Build history of the part. All positions in model axes, mm. Face numbers are marked on the shaded views. Round coordinates to 2 decimals unless told otherwise and drop trailing zeros. Order: outer loops, then holes, each group sorted by start corner. A loop starts at its lowest first (then second) coordinate and runs counter-clockwise, first axis right, second up. Notation, with made-up numbers: (-8.75, 17.5) -> (46.25, 17.5) arc R33 ccw to (46.25, 46.5) -> close; hole circle Ø9 at (81.5, -8.75). An arc over 180 degrees is marked (long way). Write item = value, one per line.
from build123d import *

# Parameters (mm, degrees)
SKETCH1_W             = 152.4
SKETCH1_H             = 101.6
BOSS_EXTRUDE2_DEPTH   = 6.35
SKETCH2_W             = 6.35
SKETCH2_H             = 12.7
SKETCH2_H_2           = 6.35
CUT_EXTRUDE2_DEPTH    = 6.35
SKETCH2_4_W           = 12.7
SKETCH2_4_H           = 6.35
CUT_EXTRUDE3_DEPTH    = 6.35
F_5_0MM_DOWEL_HOLE7_D = 5.3


with BuildPart() as part:
    # Sketch1 → Boss-Extrude2 (new body)
    with BuildSketch(Plane(origin=(0, 0, 0), x_dir=(1, 0, 0), z_dir=(0, 1, 0))):
        with Locations((76.2, 50.8)):
            Rectangle(SKETCH1_W, SKETCH1_H)
    extrude(amount=BOSS_EXTRUDE2_DEPTH)

    # Sketch2 → Cut-Extrude2 (cut)
    with BuildSketch(Plane(origin=(0, 6.35, 0), x_dir=(1, 0, 0), z_dir=(0, 1, 0))):
        with Locations((3.175, 19.05)):
            Rectangle(SKETCH2_W, SKETCH2_H)
        with Locations((3.175, 44.45)):
            Rectangle(SKETCH2_W, SKETCH2_H)
        with Locations((3.175, 69.85)):
            Rectangle(SKETCH2_W, SKETCH2_H)
        with Locations((3.175, 98.425)):
            Rectangle(SKETCH2_W, SKETCH2_H_2)
        with Locations((3.175, 92.075)):
            Rectangle(SKETCH2_W, SKETCH2_H_2)
    cut_extrude2 = extrude(amount=-CUT_EXTRUDE2_DEPTH, mode=Mode.SUBTRACT)

    # Mirror1: Cut-Extrude2 across plane
    add(cut_extrude2.mirror(Plane.ZY.offset(-76.2)), mode=Mode.SUBTRACT)

    # Sketch2_4 → Cut-Extrude3 (cut)
    with BuildSketch(Plane(origin=(0, 6.35, 0), x_dir=(1, 0, 0), z_dir=(0, 1, 0))):
        with Locations((19.05, 98.425)):
            Rectangle(SKETCH2_4_W, SKETCH2_4_H)
        with Locations((44.45, 98.425)):
            Rectangle(SKETCH2_4_W, SKETCH2_4_H)
        with Locations((69.85, 98.425)):
            Rectangle(SKETCH2_4_W, SKETCH2_4_H)
        with Locations((95.25, 98.425)):
            Rectangle(SKETCH2_4_W, SKETCH2_4_H)
        with Locations((146.05, 98.425)):
            Rectangle(SKETCH2_4_W, SKETCH2_4_H)
        with Locations((120.65, 98.425)):
            Rectangle(SKETCH2_4_W, SKETCH2_4_H)
    cut_extrude3 = extrude(amount=-CUT_EXTRUDE3_DEPTH, mode=Mode.SUBTRACT)

    # Mirror2: Cut-Extrude3 across plane
    add(cut_extrude3.mirror(Plane(origin=(0, 0, -50.8), x_dir=(1, 0, 0), z_dir=(0, 0, -1))), mode=Mode.SUBTRACT)

    # 5.0mm Dowel Hole7 (through all)
    with Locations(Plane(origin=(0, 0, 0), x_dir=(-1, 0, 0), z_dir=(0, -1, 0))):
        with Locations((-119.634, 79.65), (-32.766, 79.65), (-32.766, 21.95), (-119.634, 21.95)):
            Hole(F_5_0MM_DOWEL_HOLE7_D / 2)


solid = part.part
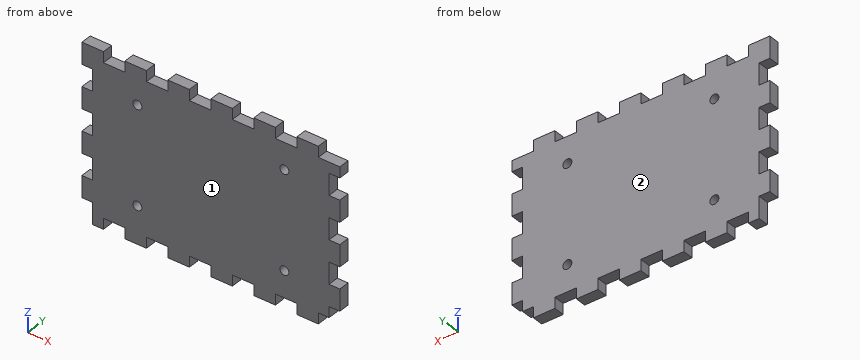
Q1. Cut at B-B, the plane z = -21.95. List the corners of the cut face in (x, y), and give its area (3 significant figures).
Check values:
outline = (6.35, 0) -> (30.12, 0) -> (30.12, 6.35) -> (6.35, 6.35) -> close; (35.42, 0) -> (116.98, 0) -> (116.98, 6.35) -> (35.42, 6.35) -> close; (122.28, 0) -> (146.05, 0) -> (146.05, 6.35) -> (122.28, 6.35) -> close
area = 820 mm²
Q2. Cut at C-C, the plane y = 5. Give the number of separate pieces and of enclosed holes in the cut face, and give its area (3 significant figures).
Check values:
separate_pieces = 1
enclosed_holes = 4
area = 13,800 mm²
Q3. Flat gauge pins, fed straight in: pin 1 (1.9 mm diameter, centred on x = 71.5, y = 4.5, fed in from +Z); pin 2 (3 mm diameter, centred on x = 119.5, y = 3.5, fed in from -Z); pin 3 (1.9 mm diameter, centred on y = 3.5, z = -97.5, fed in from -X). Where does each tip first touch, or does it go through?
Check values:
pin_1 = -6.35
pin_2 = -95.25
pin_3 = 6.35
Q4. Cut at A-A, the plane z = -79.65. List the corners of the cut face in (x, y).
Check values:
outline = (0, 0) -> (30.12, 0) -> (30.12, 6.35) -> (0, 6.35) -> close; (35.42, 0) -> (116.98, 0) -> (116.98, 6.35) -> (35.42, 6.35) -> close; (122.28, 0) -> (152.4, 0) -> (152.4, 6.35) -> (122.28, 6.35) -> close
Q5. Cut at D-D, the plane z = -69. List the corners of the cut face in (x, y), and give its area (3 significant figures).
Check values:
outline = (6.35, 0) -> (146.05, 0) -> (146.05, 6.35) -> (6.35, 6.35) -> close
area = 887 mm²
Q6. Probe probe 1 along X at (y, z) = (3.25, -79.65); probe 2 along X at (y, z) = (3, -4.5); probe 3 along X at (y, z) = (1.5, -50). List the from-to ranges inside material, lowest first.
Check values:
probe_1 = 0 to 30.12, 35.42 to 116.98, 122.28 to 152.4
probe_2 = 0 to 12.7, 25.4 to 38.1, 50.8 to 63.5, 76.2 to 88.9, 101.6 to 114.3, 127 to 139.7
probe_3 = 6.35 to 146.05
Q7. Mould opens along Y. For the marked faces 1 and 2 say: released by +Y, released by -Y, zero draft, split by the parting line, or undercut.
Check values:
face_1 = released by -Y
face_2 = released by +Y
